from build123d import *

# Parameters (mm, degrees)
SKETCH11_R                     = 3.4
SKETCH11_W                     = 3.75
SKETCH11_H                     = 3.75
T_SLOT_PROFILES_3030_2_1_DEPTH = 236


with BuildPart() as part:
    # Sketch11 → T-slot profiles 3030_2(1) (new body)
    with BuildSketch(Plane.YZ):
        with BuildLine():
            Line((-4.07, 5.6), (4.07, 5.6))
            Line((4.07, 5.6), (8.25, 9.78))
            Line((8.25, 9.78), (8.25, 13))
            Line((8.25, 13), (4.07, 13))
            Line((4.07, 13), (4.07, 15))
            Line((4.07, 15), (12.5, 15))
            ThreePointArc((12.5, 15), (14.267766953, 14.267766953), (15, 12.5))
            Line((15, 12.5), (15, 4.07))
            Line((15, 4.07), (13, 4.07))
            Line((13, 4.07), (13, 8.25))
            Line((13, 8.25), (9.78, 8.25))
            Line((9.78, 8.25), (5.6, 4.07))
            Line((5.6, 4.07), (5.6, -4.07))
            Line((5.6, -4.07), (9.78, -8.25))
            Line((9.78, -8.25), (13, -8.25))
            Line((13, -8.25), (13, -4.07))
            Line((13, -4.07), (15, -4.07))
            Line((15, -4.07), (15, -12.5))
            ThreePointArc((15, -12.5), (14.267766953, -14.267766953), (12.5, -15))
            Line((12.5, -15), (4.07, -15))
            Line((4.07, -15), (4.07, -13))
            Line((4.07, -13), (8.25, -13))
            Line((8.25, -13), (8.25, -9.78))
            Line((8.25, -9.78), (4.07, -5.6))
            Line((4.07, -5.6), (-4.07, -5.6))
            Line((-4.07, -5.6), (-8.25, -9.78))
            Line((-8.25, -9.78), (-8.25, -13))
            Line((-8.25, -13), (-4.07, -13))
            Line((-4.07, -13), (-4.07, -15))
            Line((-4.07, -15), (-12.5, -15))
            ThreePointArc((-12.5, -15), (-14.267766953, -14.267766953), (-15, -12.5))
            Line((-15, -12.5), (-15, -4.07))
            Line((-15, -4.07), (-13, -4.07))
            Line((-13, -4.07), (-13, -8.25))
            Line((-13, -8.25), (-9.78, -8.25))
            Line((-9.78, -8.25), (-5.6, -4.07))
            Line((-5.6, -4.07), (-5.6, 4.07))
            Line((-5.6, 4.07), (-9.78, 8.25))
            Line((-9.78, 8.25), (-13, 8.25))
            Line((-13, 8.25), (-13, 4.07))
            Line((-13, 4.07), (-15, 4.07))
            Line((-15, 4.07), (-15, 12.5))
            ThreePointArc((-15, 12.5), (-14.267766953, 14.267766953), (-12.5, 15))
            Line((-12.5, 15), (-4.07, 15))
            Line((-4.07, 15), (-4.07, 13))
            Line((-4.07, 13), (-8.25, 13))
            Line((-8.25, 13), (-8.25, 9.78))
            Line((-8.25, 9.78), (-4.07, 5.6))
        make_face()
        Circle(SKETCH11_R, mode=Mode.SUBTRACT)
        with Locations((11.625, 11.625)):
            Rectangle(SKETCH11_W, SKETCH11_H, mode=Mode.SUBTRACT)
        with Locations((11.625, -11.625)):
            Rectangle(SKETCH11_W, SKETCH11_H, mode=Mode.SUBTRACT)
        with Locations((-11.625, 11.625)):
            Rectangle(SKETCH11_W, SKETCH11_H, mode=Mode.SUBTRACT)
        with Locations((-11.625, -11.625)):
            Rectangle(SKETCH11_W, SKETCH11_H, mode=Mode.SUBTRACT)
    extrude(amount=T_SLOT_PROFILES_3030_2_1_DEPTH)


solid = part.part
Design review of the part built by this model. Coordinates are the model's own, in mm. A direction names the side the tool comes from. Coordinates: 2 decimals unless noted, no trailing zeros. Order: outer loops, then holes, each group sorted by start corner. A loop starts at its lowest first (then second) coordinate and runs counter-clockwise, first axis right, second up. Notation, with made-up numbers: (-29.75, 11.5) -> (24.25, 11.5) arc R6 ccw to (24.25, 22.5) -> close; hole circle Ø4 at (26.25, 52). An arc over 180 degrees is marked (long way). Use one line per item in the form item = value. Start each with the question number.
(1) Insertion check: pin 1 (8 mm diameter, centred on y = 2.5, z = 0.5, fed in from -X); pin 2 (1.6 mm diameter, centred on x = 128, y = 13.5, fed in from -Z); pin 3 (4 mm diameter, centred on x = 138, z = 0.5, fed in from -Y); pin 4 (1 mm diameter, centred on x = 66, y = -14.5, fed in from -Z). Each pin has a flat end and moves straight along its axis. Give the tip position at first contact, or say it passes through.
(2) Add section C-C on x = 207.5. Give the number of separate pieces and of enclosed holes in the cut face, plus the area to 3 significant figures.
(3) For faces 1 (the flat face through (116, 6, 13)), 2 (the flat face through (116, 0, -5.6)), 3 (the flat face through (116, -15, 8)), list the 3-axis set-ups (+Z, -Z, +X, -X, +Y, -Y) from which the entire face can be reached by the end or side of a thin tool; tool diameter is ignored.
(4) Add section A-A on z = 0. State the section outline as (x, y) points, plus the area to 3 significant figures.
(5) The part is to be moulded in two halves that separate along Z. For faces 4 (the flat face through (116, 8, -15)), 5 (the flat face through (116, 15, -8)), 6 (the flat face through (116, 12, -13.5)), say which applies: +Z half, -Z half, draft (parallel to the pull), parting line (faces both ways), or undercut.
(6) For probe 1 along Z at (x, y) = (56.5, 11.5); probe 2 along Z at (x, y) = (95.5, 0), list the stretches that pass through material, from the lowest coordinate up.
Answer block:
q1.pin_1 = 0
q1.pin_2 = -14.99
q1.pin_3 = -5.6
q1.pin_4 = -14.5
q2.separate_pieces = 1
q2.enclosed_holes = 5
q2.area = 318 mm²
q3.face_1 = +X, -X
q3.face_2 = -Z, +X, -X
q3.face_3 = +Z, -Z, +X, -X, -Y
q4.outline = (0, -5.6) -> (236, -5.6) -> (236, -3.4) -> (0, -3.4) -> close; (0, 3.4) -> (236, 3.4) -> (236, 5.6) -> (0, 5.6) -> close
q4.area = 1,040 mm²
q5.face_4 = -Z half
q5.face_5 = draft
q5.face_6 = undercut
q6.probe_1 = -15 to -13.5, -9.75 to -8.25, 8.25 to 9.75, 13.5 to 15
q6.probe_2 = -5.6 to -3.4, 3.4 to 5.6
